Geometry check sheet. Reference: the model listing, model coordinates, mm. Face numbers are marked on the shaded views. A direction names the side the tool comes from. Coordinates: 2 decimals unless noted, no trailing zeros. Write each loop counter-clockwise with the first axis right and the second up, starting at its lowest first coordinate (ties: lowest second). Pieces come first, ordered by that corner, then holes. Notation, with made-up numbers: M 61.25,81.5 L 95.25,81.5 A13 ccw 95.25,88.5 Z; hole C -27,15 d7. An arc over 180 degrees is marked long. Put each result on its own line as item: value. Start each with the question number.
1) Mould release check, pull along Z, two halves, no side actions. Record for the marked faces 4, 5 and 6: released by +Z, released by -Z, zero draft, split by the parting line, or undercut.
2) Cross-section at A-A on x = 1. Record the cut outline in (y, z), plus the area to 3 significant figures.
3) Gauge pin test, flat ends, axial feed: pin 1 (6 mm diameter, centred on x = 5.5, z = -2, fed in from -Y); pin 2 (1.2 mm diameter, centred on x = 8.5, y = 3.5, fed in from -Z); pin 3 (2 mm diameter, centred on y = 2.5, z = 6.5, fed in from +X); pin 4 (6 mm diameter, centred on y = 5, z = -2.5, fed in from +X). Record the tip position at first contact, or that the pin passes through.
4) Scan lines: line 1 along Z through (x, y) = (-4.5, 2.5); line 2 along X through (y, z) = (4.5, 1.5); line 3 along X through (y, z) = (5.25, 8.5). Record each from-to range of solid material in increasing order.
5) Set-up check for the marked faces 1, 2 and 3: record each of +Z, -Z, +X, -X, +Y, -Y from which the full face is reachable in a straight line by a thin tool's end or side.
6) Cross-section at D-D on z = -3.25. Record the cut outline in (x, y).
7) Cross-section at B-B on x = -2.5. Record the cut outline in (y, z), plus the area to 3 significant figures.
8) Cross-section at C-C on y = 5.25. Record the cut outline in (x, z), plus the area to 3 significant figures.
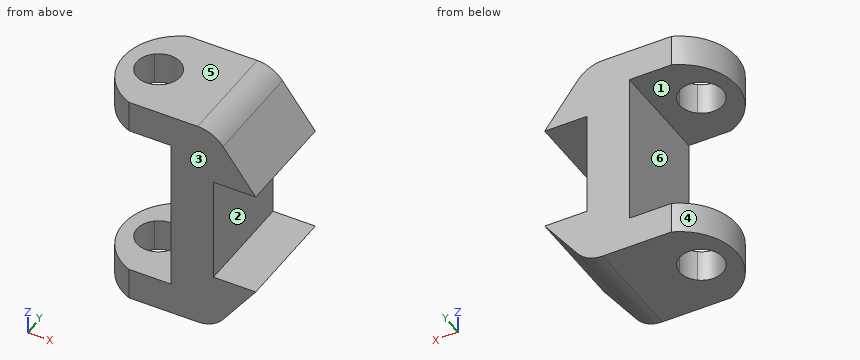
from build123d import *

# Parameters (mm, degrees)
BOSS_EXTRUDE1_DEPTH     = 10
CUT_EXTRUDE1_DEPTH      = 22.113029153
CUT_EXTRUDE1_DEPTH_BACK = 22.113029153
BOSS_EXTRUDE2_DEPTH     = 10
FILLET1_R               = 3
CUT_EXTRUDE2_DEPTH      = 25.987196722
CUT_EXTRUDE2_DEPTH_BACK = 25.987196722


with BuildPart() as part:
    # Sketch1 → Boss-Extrude1 (new body)
    with BuildSketch(Plane(origin=(0, 0, 0), x_dir=(1, 0, 0), z_dir=(0, 1, 0))):
        Polygon((-6, -10.3), (6, -10.3), (6, 10.3), (-6, 10.3), (-6, 7.3), (2, 7.3), (2, -7.3), (-6, -7.3), align=None)
    extrude(amount=BOSS_EXTRUDE1_DEPTH)

    # Sketch2 → Cut-Extrude1 (cut, two sides: drawn at the far end of the back side and taken through both)
    with BuildSketch(Plane.XY.offset(-7.3).offset(-CUT_EXTRUDE1_DEPTH_BACK)):
        with BuildLine():
            ThreePointArc((-3.280624847, 6.600781059), (-3.600781059, 3.719375153), (-0.719375153, 3.399218941))
            Line((-0.719375153, 3.399218941), (-3.280624847, 6.600781059))
        make_face()
        with BuildLine():
            Line((-3.280624847, 6.600781059), (-0.719375153, 3.399218941))
            ThreePointArc((-0.719375153, 3.399218941), (-0.152328366, 4.111963102), (0.05, 5))
            ThreePointArc((0.05, 5), (-1.111963102, 6.847671634), (-3.280624847, 6.600781059))
        make_face()
    extrude(amount=CUT_EXTRUDE1_DEPTH + CUT_EXTRUDE1_DEPTH_BACK, mode=Mode.SUBTRACT)

    # Sketch3 → Boss-Extrude2 (add)
    with BuildSketch(Plane(origin=(0, 10, 0), x_dir=(1, 0, 0), z_dir=(0, 1, 0))):
        Polygon((10, 5), (6, 10.3), (6, 5), align=None)
        Polygon((6, -10.3), (10, -5), (6, -5), align=None)
    extrude(amount=-BOSS_EXTRUDE2_DEPTH)

    # Fillet1
    fillet1_edges = [part.edges().sort_by_distance(p)[0] for p in [
        (6, 5, -10.3),
        (6, 5, 10.3),
    ]]
    fillet(fillet1_edges, radius=FILLET1_R)

    # Sketch4 → Cut-Extrude2 (cut, two sides: drawn at the far end of the back side and taken through both)
    with BuildSketch(Plane(origin=(0, 0, -10.3), x_dir=(-1, 0, 0), z_dir=(0, 0, -1)).offset(-CUT_EXTRUDE2_DEPTH_BACK)):
        with BuildLine():
            Line((2, 10), (6, 10))
            Line((6, 10), (6, 0))
            Line((6, 0), (2, 0))
            ThreePointArc((2, 0), (5.353933752, 5), (2, 10))
        make_face()
    extrude(amount=CUT_EXTRUDE2_DEPTH + CUT_EXTRUDE2_DEPTH_BACK, mode=Mode.SUBTRACT)


solid = part.part
Answer key:
1. face 4: zero draft
1. face 5: released by +Z
1. face 6: undercut
2. outline: M 0,-10.3 L 10,-10.3 L 10,-7.3 L 0,-7.3 Z; M 0,7.3 L 10,7.3 L 10,10.3 L 0,10.3 Z
2. area: 60.0 mm²
3. pin 1: stops at y = 0
3. pin 2: stops at z = -7.78
3. pin 3: stops at x = 9.62
3. pin 4: stops at x = 10
4. line 1: z = -10.3 to -7.3, 7.3 to 10.3
4. line 2: x = 2 to 6
4. line 3: x = -5.35 to -4.03, 0.03 to 7.36
5. face 1: -X, +Y, -Y
5. face 2: +X, +Y, -Y
5. face 3: +Z, -Z, +X, -X, -Y
6. outline: M 2,0 L 6,0 L 6,10 L 2,10 Z
7. outline: M 0.24,-10.3 L 3.01,-10.3 L 3.01,-7.3 L 0.24,-7.3 Z; M 0.24,7.3 L 3.01,7.3 L 3.01,10.3 L 0.24,10.3 Z; M 6.99,-10.3 L 9.76,-10.3 L 9.76,-7.3 L 6.99,-7.3 Z; M 6.99,7.3 L 9.76,7.3 L 9.76,10.3 L 6.99,10.3 Z
7. area: 33.3 mm²
8. outline: M -5.35,-10.3 L -4.03,-10.3 L -4.03,-7.3 L -5.35,-7.3 Z; M -5.35,7.3 L -4.03,7.3 L -4.03,10.3 L -5.35,10.3 Z; M 0.03,-10.3 L 4.51,-10.3 A3 ccw 6.9,-9.11 L 10,-5 L 6,-5 L 6,5 L 10,5 L 6.9,9.11 A3 ccw 4.51,10.3 L 0.03,10.3 L 0.03,7.3 L 2,7.3 L 2,-7.3 L 0.03,-7.3 Z
8. area: 123 mm²
